from build123d import *

# Parameters (mm, degrees)
BOSS_EXTRUDE1_DEPTH = 4
BOSS_EXTRUDE1_TAPER = 10
CUT_EXTRUDE1_START  = 4
SKETCH1_3_R         = 1.1
CUT_EXTRUDE1_DEPTH  = 4
CUT_EXTRUDE2_START  = 4
SKETCH1_4_R         = 8.4
SKETCH1_4_R_2       = 1.1
CUT_EXTRUDE2_DEPTH  = 3


with BuildPart() as part:
    # Sketch1 → Boss-Extrude1 (new body)
    with BuildSketch(Plane(origin=(0, 0, 0), x_dir=(1, 0, 0), z_dir=(0, 1, 0))):
        with BuildLine():
            ThreePointArc((-29.7, 28.547302995), (-35.4, 27.019992598), (-39.572689603, 22.847302995))
            Line((-39.572689603, 22.847302995), (-49.472689603, 5.7))
            ThreePointArc((-49.472689603, 5.7), (-51, 0), (-49.472689603, -5.7))
            Line((-49.472689603, -5.7), (-39.572689603, -22.847302995))
            ThreePointArc((-39.572689603, -22.847302995), (-35.4, -27.019992598), (-29.7, -28.547302995))
            Line((-29.7, -28.547302995), (-9.9, -28.547302995))
            ThreePointArc((-9.9, -28.547302995), (-4.2, -27.019992598), (-0.027310397, -22.847302995))
            Line((-0.027310397, -22.847302995), (9.872689603, -5.7))
            ThreePointArc((9.872689603, -5.7), (11.4, 0), (9.872689603, 5.7))
            Line((9.872689603, 5.7), (-0.027310397, 22.847302995))
            ThreePointArc((-0.027310397, 22.847302995), (-4.2, 27.019992598), (-9.9, 28.547302995))
            Line((-9.9, 28.547302995), (-29.7, 28.547302995))
        make_face()
    extrude(amount=BOSS_EXTRUDE1_DEPTH, taper=BOSS_EXTRUDE1_TAPER)

    # Sketch1<3> → Cut-Extrude1 (cut)
    with BuildSketch(Plane(origin=(0, 0, 0), x_dir=(1, 0, 0), z_dir=(0, 1, 0)).offset(CUT_EXTRUDE1_START)):
        with Locations(Location((-9.9, -17.147302995, 0), (0, 0, 270))):
            Circle(SKETCH1_3_R)
        with Locations(Location((0, 0, 0), (0, 0, 270))):
            Circle(SKETCH1_3_R)
        with Locations(Location((-29.7, -17.147302995, 0), (0, 0, 270))):
            Circle(SKETCH1_3_R)
        with Locations(Location((-39.6, 0, 0), (0, 0, 270))):
            Circle(SKETCH1_3_R)
        with Locations(Location((-9.9, 17.147302995, 0), (0, 0, 270))):
            Circle(SKETCH1_3_R)
        with Locations(Location((-29.7, 17.147302995, 0), (0, 0, 270))):
            Circle(SKETCH1_3_R)
        with Locations(Location((-19.8, 0, 0), (0, 0, 270))):
            Circle(SKETCH1_3_R)
    extrude(amount=-CUT_EXTRUDE1_DEPTH, mode=Mode.SUBTRACT)

    # Sketch1<4> → Cut-Extrude2 (cut)
    # profile 1 of 6: a face of its own
    with BuildSketch(Plane(origin=(0, 0, 0), x_dir=(1, 0, 0), z_dir=(0, 1, 0)).offset(CUT_EXTRUDE2_START)):
        with Locations(Location((0, 0, 0), (0, 0, 270))):
            Circle(SKETCH1_4_R)
        with Locations(Location((0, 0, 0), (0, 0, 270))):
            Circle(SKETCH1_4_R_2, mode=Mode.SUBTRACT)
    # profile 2 of 6: a face of its own
    with BuildSketch(Plane(origin=(0, 0, 0), x_dir=(1, 0, 0), z_dir=(0, 1, 0)).offset(CUT_EXTRUDE2_START)):
        with BuildLine():
            Line((-29.7, -25.547302995), (-9.9, -25.547302995))
            ThreePointArc((-9.9, -25.547302995), (-1.786223222, -14.97322241), (-14.100001087, -9.872690231))
            ThreePointArc((-14.100001087, -9.872690231), (-16.822981756, -11.004424673), (-19.745150662, -11.39986805))
            ThreePointArc((-19.745150662, -11.39986805), (-19.772689603, -11.447302995), (-19.8, -11.494869891))
            ThreePointArc((-19.8, -11.494869891), (-19.827310397, -11.447302995), (-19.854849338, -11.39986805))
            ThreePointArc((-19.854849338, -11.39986805), (-22.777018876, -11.004424502), (-25.500000049, -9.872689575))
            ThreePointArc((-25.500000049, -9.872689575), (-37.813776948, -14.973223043), (-29.7, -25.547302995))
        make_face()
        with Locations(Location((-9.9, -17.147302995, 0), (0, 0, 270))):
            Circle(SKETCH1_4_R_2, mode=Mode.SUBTRACT)
        with Locations(Location((-29.7, -17.147302995, 0), (0, 0, 270))):
            Circle(SKETCH1_4_R_2, mode=Mode.SUBTRACT)
    # profile 3 of 6: a face of its own
    with BuildSketch(Plane(origin=(0, 0, 0), x_dir=(1, 0, 0), z_dir=(0, 1, 0)).offset(CUT_EXTRUDE2_START)):
        with Locations(Location((-9.9, 17.147302995, 0), (0, 0, 270))):
            Circle(SKETCH1_4_R)
        with Locations(Location((-9.9, 17.147302995, 0), (0, 0, 270))):
            Circle(SKETCH1_4_R_2, mode=Mode.SUBTRACT)
    # profile 4 of 6: a face of its own
    with BuildSketch(Plane(origin=(0, 0, 0), x_dir=(1, 0, 0), z_dir=(0, 1, 0)).offset(CUT_EXTRUDE2_START)):
        with Locations(Location((-19.8, 0, 0), (0, 0, 270))):
            Circle(SKETCH1_4_R)
        with Locations(Location((-19.8, 0, 0), (0, 0, 270))):
            Circle(SKETCH1_4_R_2, mode=Mode.SUBTRACT)
    # profile 5 of 6: a face of its own
    with BuildSketch(Plane(origin=(0, 0, 0), x_dir=(1, 0, 0), z_dir=(0, 1, 0)).offset(CUT_EXTRUDE2_START)):
        with Locations(Location((-39.6, 0, 0), (0, 0, 270))):
            Circle(SKETCH1_4_R)
        with Locations(Location((-39.6, 0, 0), (0, 0, 270))):
            Circle(SKETCH1_4_R_2, mode=Mode.SUBTRACT)
    # profile 6 of 6: a face of its own
    with BuildSketch(Plane(origin=(0, 0, 0), x_dir=(1, 0, 0), z_dir=(0, 1, 0)).offset(CUT_EXTRUDE2_START)):
        with Locations(Location((-29.7, 17.147302995, 0), (0, 0, 270))):
            Circle(SKETCH1_4_R)
        with Locations(Location((-29.7, 17.147302995, 0), (0, 0, 270))):
            Circle(SKETCH1_4_R_2, mode=Mode.SUBTRACT)
    extrude(amount=-CUT_EXTRUDE2_DEPTH, mode=Mode.SUBTRACT)


solid = part.part
Verification items for the finished model (mm, model axes). A direction names the side the tool comes from. Give positions to 0.01 mm unless a question says otherwise; leave off trailing zeros. Write each loop counter-clockwise with the first axis right and the second up, starting at its lowest first coordinate (ties: lowest second). Pieces come first, ordered by that corner, then holes. Notation, with made-up numbers: (8, 48) - (26, 48) arc R30 ccw to (26, 86) - close; hole circle Ø11 at (-14, 29.25). An arc over 180 degrees is marked (long way). Answer as CSV lines item,"result". Start each with the question number.
1. Depth check by flat-ended pin: pin 1 (1.5 mm diameter, centred on y = 2.5, z = 6, fed in from -X); pin 2 (5 mm diameter, centred on x = -20.5, z = 16, fed in from +Y); pin 3 (1.5 mm diameter, centred on y = 1, z = 21.5, fed in from -X); pin 4 (1.8 mm diameter, centred on x = -39.6, z = 0, fed in from -Y). Enter the tip coordinate at first touch or a pass-through.
2. Draft check along Z on faces 3 (the face through (-7.377, 2.521, -9.135)), 4 (the face through (-24, 4, -8)), 5 (the face through (-50.64, 2.03, -0.08)). Enter one of: pulls with the +Z half, pulls with the -Z half, needs draft (parallel to the pull), parting line crosses it, or undercut.
3. Thickness scan on line 1 (X direction, y = 2.8, z = -12); line 2 (X direction, y = 3.3, z = -4.5); line 3 (Z direction, x = -27.5, y = 3.1). Record the ranges inside material, lowest first.
4. Sectioned sample at B-B (y = 2.3). Count the separate pieces of the cut face and the enclosed holes in it, then the cut area to 3 significant figures.
5. Sectioned sample at A-A (z = 0). Record the boundary of the cut face in (x, y).
6. Set-up check for faces 1 (the face through (-1.733, 2.521, 15.182)), 2 (the face through (-10.6, 0.5, 16.3)): record each of +Z, -Z, +X, -X, +Y, -Y from which the full face is reachable in a straight line by a thin tool's end or side.
Derived:
1,pin 1,"x = -49.25"
1,pin 2,"y = 1"
1,pin 3,"x = -40.61"
1,pin 4,"through"
2,face 3,"undercut"
2,face 4,"needs draft"
2,face 5,"parting line crosses it"
3,line 1,"-45.27 to -36.34, -23.06 to -16.54, -3.26 to 5.67"
3,line 2,"-49.44 to -46.69, -32.51 to -26.89, -12.71 to -7.09, 7.09 to 9.84"
3,line 3,"-28 to -25.25, -9.04 to -3.36, 3.36 to 9.04, 25.55 to 28"
4,separate pieces,"1"
4,enclosed holes,"6"
4,area,"1,070 mm²"
5,outline,"(-51, 0) - (-40.7, 0) - (-40.7, 1) - (-48, 1) - (-48, 4) - (-50.29, 4) - close; (-38.5, 0) - (-20.9, 0) - (-20.9, 1) - (-28.2, 1) - (-28.2, 4) - (-31.2, 4) - (-31.2, 1) - (-38.5, 1) - close; (-18.7, 0) - (-1.1, 0) - (-1.1, 1) - (-8.4, 1) - (-8.4, 4) - (-11.4, 4) - (-11.4, 1) - (-18.7, 1) - close; (1.1, 0) - (11.4, 0) - (10.69, 4) - (8.4, 4) - (8.4, 1) - (1.1, 1) - close"
6,face 1,"+Y"
6,face 2,"+Y, -Y"
